from build123d import *

# Parameters (mm, degrees)
BOSS_EXTRUDE2_DEPTH      = 2
BOSS_EXTRUDE2_DEPTH_BACK = 7
SKETCH2_R                = 12.45
SKETCH3_R                = 1.475
CUT_EXTRUDE1_DEPTH       = 6.05
SKETCH4_R                = 7
CUT_EXTRUDE2_DEPTH       = 4.05


with BuildPart() as part:
    # Sketch2 → Boss-Extrude2 (new, two sides: drawn at the far end of the back side and taken through both)
    with BuildSketch(Plane(origin=(0, 14, 0), x_dir=(1, 0, 0), z_dir=(0, 1, 0)).offset(-BOSS_EXTRUDE2_DEPTH_BACK)):
        with Locations(Location((-0.498, 0, 0), (0, 0, 270))):
            Circle(SKETCH2_R)
    extrude(amount=BOSS_EXTRUDE2_DEPTH + BOSS_EXTRUDE2_DEPTH_BACK)

    # Sketch3 → Cut-Extrude1 (cut)
    with BuildSketch(Plane.XZ.offset(-7)):
        with Locations(Location((9.5, 0, 0), (0, 0, 270))):
            Circle(SKETCH3_R)
        with Locations(Location((4.5, -8.660254038, 0), (0, 0, 270))):
            Circle(SKETCH3_R)
        with Locations(Location((-5.5, -8.660254038, 0), (0, 0, 270))):
            Circle(SKETCH3_R)
        with Locations(Location((-10.5, 0, 0), (0, 0, 270))):
            Circle(SKETCH3_R)
        with Locations(Location((-5.5, 8.660254038, 0), (0, 0, 270))):
            Circle(SKETCH3_R)
        with Locations(Location((4.5, 8.660254038, 0), (0, 0, 270))):
            Circle(SKETCH3_R)
    extrude(amount=-CUT_EXTRUDE1_DEPTH, mode=Mode.SUBTRACT)

    # Sketch4 → Cut-Extrude2 (cut)
    with BuildSketch(Plane.XZ.offset(-7)):
        with Locations(Location((-0.5, 0, 0), (0, 0, 270))):
            Circle(SKETCH4_R)
    extrude(amount=-CUT_EXTRUDE2_DEPTH, mode=Mode.SUBTRACT)


solid = part.part
Model file for the job. Use its own axes, mm. A direction names the side the tool comes from. Give positions to 0.01 mm unless a question says otherwise; leave off trailing zeros. Loops run counter-clockwise (first coordinate to the right, second up) from the corner with the lowest first, then second, coordinate; pieces in that order, holes last.
1) Flat gauge pins, fed straight in: pin 1 Ø2.5 at (x, z) = (-5.5, 8.66) entering from -Y; pin 2 Ø1.5 at (x, y) = (5.5, 13) entering from +Z; pin 3 Ø8 at (x, z) = (-0.5, -3.5) entering from -Y. Where does each tip first touch, or does it go through?
2) Wall check: line 1 (X direction, y = 8.75, z = 0) (3 decimals); line 2 (X direction, y = 8, z = -7.5); line 3 (X direction, y = 11, z = 0.75). Give the ranges that are in metal, low to high.
3) Saw through at C-C (z = 5.25). Write the cut outline in (x, y), plus the area to 3 significant figures.
4) Tool access for faces 1 (the flat face through (-6, 7, 5)), 2 (the cylindrical face through (-9.256, 9.983, -0.793)): list every direction of +Z, -Z, +X, -X, +Y, -Y with a clear straight run to the whole face (end or side of a thin tool).
5) Saw through at B-B (x = -10.5). Write the cut outline in (y, z) (3 decimals), plus the area to 3 significant figures.
6) Saw through at D-D (z = 1). Write the cut outline in (x, y), plus the area to 3 significant figures.
7) Saw through at A-A (y = 11.75). Write the cut outline in (x, z) (3 decimals).
8) Pull direction X, two halves, no side cores. Call faces 3 (the flat face through (0, 16, 0)), 4 (the cylindrical face through (10.744, 9.983, -0.793)), 5 (the cylindrical face through (7.916, 11.437, -9.176)): +X half, -X half, draft (parallel to the pull), parting line (faces both ways), or undercut.
Answer block:
1. pin 1: stops at y = 13.05
1. pin 2: stops at z = 11.29
1. pin 3: stops at y = 7
2. line 1: x = -12.948 to -11.975, -9.025 to -7.5, 6.5 to 8.025, 10.975 to 11.952
2. line 2: x = -10.44 to -6.41, -4.59 to 3.59, 5.41 to 9.44
2. line 3: x = -12.93 to -11.77, -9.23 to -7.46, 6.46 to 8.23, 10.77 to 11.93
3. outline: (-11.79, 7) - (-5.13, 7) - (-5.13, 11.05) - (4.13, 11.05) - (4.13, 7) - (10.79, 7) - (10.79, 16) - (-11.79, 16) - close
3. area: 166 mm2
4. face 1: +Z, -Z, +X, -X, -Y
4. face 2: -Y
5. outline: (7, -7.414) - (16, -7.414) - (16, 7.414) - (7, 7.414) - (7, 1.475) - (13.05, 1.475) - (13.05, -1.475) - (7, -1.475) - close
5. area: 116 mm2
6. outline: (-12.91, 7) - (-11.58, 7) - (-11.58, 13.05) - (-9.42, 13.05) - (-9.42, 7) - (-7.43, 7) - (-7.43, 11.05) - (6.43, 11.05) - (6.43, 7) - (8.42, 7) - (8.42, 13.05) - (10.58, 13.05) - (10.58, 7) - (11.91, 7) - (11.91, 16) - (-12.91, 16) - close
6. area: 141 mm2
7. outline: circle Ø24.9 at (-0.498, 0); hole circle Ø2.95 at (-10.5, 0); hole circle Ø2.95 at (-5.5, -8.66); hole circle Ø2.95 at (-5.5, 8.66); hole circle Ø2.95 at (4.5, -8.66); hole circle Ø2.95 at (4.5, 8.66); hole circle Ø2.95 at (9.5, 0)
8. face 3: draft
8. face 4: undercut
8. face 5: parting line
